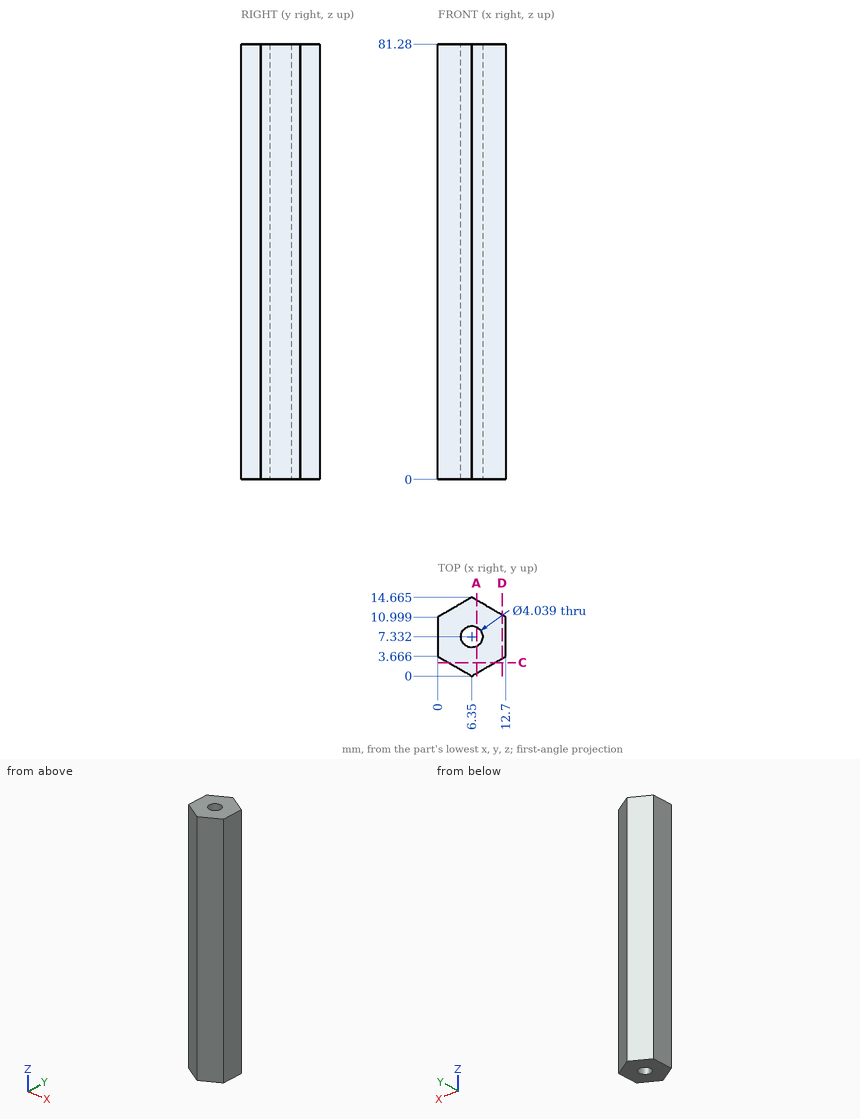
For this review, use the dimensioned drawing (mm, ordinates from the lowest corner) and the shaded views. Round coordinates to 2 decimals unless told otherwise and drop trailing zeros. Write each loop counter-clockwise with the first axis right and the second up, starting at its lowest first coordinate (ties: lowest second). Pieces come first, ordered by that corner, then holes. Notation, with made-up numbers: (-22, 55.25) - (22, 55.25) arc R13 cw to (22, 75.25) - close; hole circle Ø3 at (72.25, -5). An arc over 180 degrees is marked (long way). Use CSV: the item, a comma, the result in double quotes.
1) Clearance check with flat-ended pins moving along their axes: pin 1 Ø3 at (x, z) = (4, 39) entering from +Y (1 decimal); pin 2 Ø3.5 at (x, y) = (6.35, 7.33) entering from -Z; pin 3 Ø1.5 at (y, z) = (3, 50.5) entering from +X; pin 4 Ø1 at (x, z) = (2, 68) entering from -Y. State where each tip first meets the part, or that it passes through.
Conclusion:
pin 1,"stops at y = 14.2"
pin 2,"passes through"
pin 3,"stops at x = 12.7"
pin 4,"stops at y = 2.22"
2) Add section A-A on x = 7.25. Write out the cut boundary in (y, z) (1 decimal).
Conclusion:
outline,"(0.5, 0) - (5.5, 0) - (5.5, 81.3) - (0.5, 81.3) - close; (9.1, 0) - (14.1, 0) - (14.1, 81.3) - (9.1, 81.3) - close"
3) Wall thickness on line 1 along Y through (x, z) = (7, 61.5) (1 decimal); line 2 along Y through (x, z) = (4.75, 36) (1 decimal); line 3 along X through (y, z) = (5.75, 51) (1 decimal): over which ranges is each line inside the solid? List them lowest first. Write a range as from..to.
Conclusion:
line 1,"y = 0.4..5.4, 9.2..14.3"
line 2,"y = 0.9..6.1, 8.6..13.7"
line 3,"x = 0..5.1, 7.6..12.7"
4) Add section C-C on y = 2.5. Write out the cut boundary in (x, z), and give its area (3 significant figures).
Conclusion:
outline,"(2.02, 0) - (10.68, 0) - (10.68, 81.28) - (2.02, 81.28) - close"
area,"704 mm^2"
5) Add section D-D on x = 12. Write out the cut boundary in (y, z).
Conclusion:
outline,"(3.26, 0) - (11.4, 0) - (11.4, 81.28) - (3.26, 81.28) - close"
